Source: three-view drawing plus pictorial views. Frame: mm from the lowest corner of the part. A direction names the side the tool comes from. Round coordinates to 2 decimals unless told otherwise and drop trailing zeros. Loops run counter-clockwise (first coordinate to the right, second up) from the corner with the lowest first, then second, coordinate; pieces in that order, holes last. Notation, with made-up numbers: (84.25, 83) -> (95.25, 83) arc R29 cw to (95.25, 121) -> close; hole circle Ø9 at (-13.5, 75.5). An arc over 180 degrees is marked (long way). Answer in a Markdown table with one row per item.
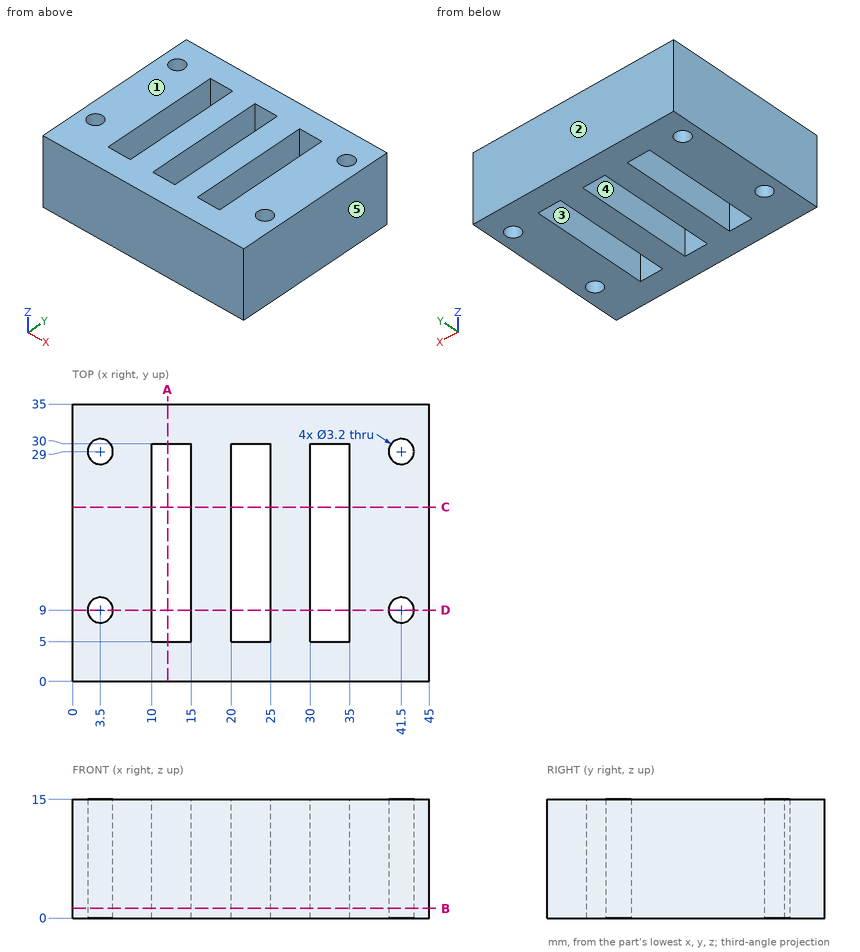
Item 1: Cut plane B-B (z = 1.25). Output: boundary loops of the cut face in (x, y), then the cut area to 3 significant figures.
Answer:
| item | result |
|---|---|
| outline | (0, 0) -> (45, 0) -> (45, 35) -> (0, 35) -> close; hole circle Ø3.2 at (3.5, 9); hole circle Ø3.2 at (3.5, 29); hole (10, 5) -> (15, 5) -> (15, 30) -> (10, 30) -> close; hole (20, 5) -> (25, 5) -> (25, 30) -> (20, 30) -> close; hole (30, 5) -> (35, 5) -> (35, 30) -> (30, 30) -> close; hole circle Ø3.2 at (41.5, 9); hole circle Ø3.2 at (41.5, 29) |
| area | 1,170 mm² |
Item 2: Cut plane A-A (x = 12). Output: boundary loops of the cut face in (y, z).
Answer:
| item | result |
|---|---|
| outline | (0, 0) -> (5, 0) -> (5, 15) -> (0, 15) -> close; (30, 0) -> (35, 0) -> (35, 15) -> (30, 15) -> close |
Item 3: Reachability of the marked faces 4 and 5 from +Z, -Z, +X, -X, +Y, -Y: full face, straight path, thin tool, end or side. Return the list, or none.
Answer:
| item | result |
|---|---|
| face 4 | +Z, -Z |
| face 5 | +Z, -Z, +X, +Y, -Y |
Item 4: Draft query along Y for the marked faces 1, 2 and 3. Return one class per face: pulls with the +Y half, pulls with the -Y half, needs draft (parallel to the pull), parting line crosses it, or undercut.
Answer:
| item | result |
|---|---|
| face 1 | needs draft |
| face 2 | pulls with the +Y half |
| face 3 | undercut |
Item 5: Cut plane C-C (y = 22). Output: boundary loops of the cut face in (x, z), then the cut area to 3 significant figures.
Answer:
| item | result |
|---|---|
| outline | (0, 0) -> (10, 0) -> (10, 15) -> (0, 15) -> close; (15, 0) -> (20, 0) -> (20, 15) -> (15, 15) -> close; (25, 0) -> (30, 0) -> (30, 15) -> (25, 15) -> close; (35, 0) -> (45, 0) -> (45, 15) -> (35, 15) -> close |
| area | 450 mm² |
Item 6: Cut plane D-D (y = 9). Output: boundary loops of the cut face in (x, z).
Answer:
| item | result |
|---|---|
| outline | (0, 0) -> (1.9, 0) -> (1.9, 15) -> (0, 15) -> close; (5.1, 0) -> (10, 0) -> (10, 15) -> (5.1, 15) -> close; (15, 0) -> (20, 0) -> (20, 15) -> (15, 15) -> close; (25, 0) -> (30, 0) -> (30, 15) -> (25, 15) -> close; (35, 0) -> (39.9, 0) -> (39.9, 15) -> (35, 15) -> close; (43.1, 0) -> (45, 0) -> (45, 15) -> (43.1, 15) -> close |
Item 7: Line query: probe 1 along Y at (x, z) = (41.5, 8.25); probe 2 along Y at (x, z) = (4, 13.5); probe 3 along Y at (x, z) = (10.5, 11.5). Output: solid intervals per line, ascending. Write a range as [from, to].
Answer:
| item | result |
|---|---|
| probe 1 | y = [0, 7.4], [10.6, 27.4], [30.6, 35] |
| probe 2 | y = [0, 7.48], [10.52, 27.48], [30.52, 35] |
| probe 3 | y = [0, 5], [30, 35] |
